Work out the finished part from the listing and answer in its coordinate system (mm). A direction names the side the tool comes from. Coordinates: 2 decimals unless noted, no trailing zeros. Order: outer loops, then holes, each group sorted by start corner. A loop starts at its lowest first (then second) coordinate and runs counter-clockwise, first axis right, second up. Notation, with made-up numbers: (45, 80.25) -> (75, 80.25) arc R25 ccw to (75, 116.25) -> close; hole circle Ø7 at (87.5, -18). An arc over 180 degrees is marked (long way). Write item = value, one per line. Start each with the question number.
Q1. The part is cut by section D-D, the plane y = 50. Determine the outline of the cut face in (x, z).
Q2. Straight lines are drawn through the part: L1, parallel to Y at x = -3.75, z = 0; L2, parallel to Y at x = 10.25, z = 3; L3, parallel to Y at x = -2, z = 58. For each, find the intervals that lie inside material, in ascending order. Write a range as from..to.
Q3. The part is cut by section B-B, the plane z = -32. Determine the outline of the cut face in (x, y), plus the area to 3 significant figures.
Q4. Flat-ended cylindrical pins translate along their axes: pin 1 (12 mm diameter, centred on x = -6, z = 62.5, fed in from -Y); pin 2 (8 mm diameter, centred on x = 3, z = 39.5, fed in from +Y); pin 3 (1 mm diameter, centred on x = -4.5, y = -39, fed in from +Z); pin 4 (12 mm diameter, centred on x = 4.5, y = -254.5, fed in from -Z). Find the tip coordinate at first contact, or state that the pin passes through.
Q5. For a pull along Y with two mould halves and no side action, classify faces 1 (the flat face through (0, -325, 0)), 2 (the flat face through (0, 325, 0)), 3 (the cylindrical face through (6.72, -169.12, -10.54)) as +Y half, -Y half, draft (parallel to the pull), parting line (faces both ways), or undercut.
Q6. The part is cut by section C-C, the plane y = -174. Determine the outline of the cut face in (x, z).
Q7. The part is cut by section A-A, the plane z = 80. Determine the outline of the cut face in (x, y), plus the area to 3 significant figures.
Q8. Which of the six approach directions +Z, -Z, +X, -X, +Y, -Y give full straight-line access (tool end or side, diameter ignored) to faces 4 (the cylindrical face through (-2.71, -306.195, 12.203)), 5 (the cylindrical face through (-1.627, 306.86, -12.394)), 6 (the cylindrical face through (-1.627, 85.665, -92.394))?
```python
from build123d import *

# Parameters (mm, degrees)
F2_R = 12.5


with BuildPart() as f3:
    # F3: sweep along a path in F0
    with BuildLine(Plane.YZ) as f3_path:
        Line((-325, 0), (-290, 0))
        Line((-290, 0), (-290, -80))
        Line((-290, -80), (-220, -80))
        Line((-220, -80), (-220, 0))
        Line((-220, 0), (-120, 0))
        Line((-120, 0), (-120, 80))
        Line((-120, 80), (-50, 80))
        Line((-50, 80), (-50, 0))
        Line((-50, 0), (50, 0))
        Line((50, 0), (50, -80))
        Line((50, -80), (120, -80))
        Line((120, -80), (120, 0))
        Line((120, 0), (220, 0))
        Line((220, 0), (220, 80))
        Line((220, 80), (290, 80))
        Line((290, 80), (290, 0))
        Line((290, 0), (325, 0))
    # F2 (on plane+point) → F3 (sweep)
    with BuildSketch(Plane.XZ.offset(325)):
        Circle(F2_R)
    sweep(path=f3_path.line, transition=Transition.RIGHT)


solid = f3.part
```
Model answer:
q1.outline = (-12.5, -80) arc R12.5 ccw to (12.5, -80) -> (12.5, 0) arc R12.5 ccw to (-12.5, 0) -> close
q2.L1 = -325..-278.08, -231.92..-108.08, -61.92..61.92, 108.08..231.92, 278.08..325
q2.L2 = -325..-282.85, -227.15..-112.85, -57.15..57.15, 112.85..227.15, 282.85..325
q2.L3 = -132.34..-107.66, -62.34..-37.66, 207.66..232.34, 277.66..302.34
q3.outline = circle Ø25 at (0, -290); circle Ø25 at (0, -220); circle Ø25 at (0, 50); circle Ø25 at (0, 120)
q3.area = 1,960 mm2
q4.pin_1 = -132.5
q4.pin_2 = 302.5
q4.pin_3 = 91.84
q4.pin_4 = -92.5
q5.face_1 = -Y half
q5.face_2 = +Y half
q5.face_3 = undercut
q6.outline = circle Ø25 at (0, 0)
q7.outline = (-12.5, -120) arc R12.5 ccw to (12.5, -120) -> (12.5, -50) arc R12.5 ccw to (-12.5, -50) -> close; (-12.5, 220) arc R12.5 ccw to (12.5, 220) -> (12.5, 290) arc R12.5 ccw to (-12.5, 290) -> close
q7.area = 4,480 mm2
q8.face_4 = -Y
q8.face_5 = +Y
q8.face_6 = none
